from build123d import *

# Parameters (mm, degrees)
ESBO_O1_R                = 2.5
ESBO_O1_R_2              = 7.5
RESSALTO_EXTRUS_O1_DEPTH = 3


with BuildPart() as part:
    # Esboço1 → Ressalto-extrusão1 (new body)
    with BuildSketch(Plane.XY):
        Polygon((40.700385396, -30), (10.700385396, -30), (10.700385396, -33), (-19.299614604, -33), (-19.299614604, -30), (-49.299614604, -30), (-49.299614604, -33), (-79.299614604, -33), (-79.299614604, -30), (-82.299614604, -30), (-82.299614604, -18), (-79.299614604, -18), (-79.299614604, -6), (-82.299614604, -6), (-82.299614604, 6), (-79.299614604, 6), (-79.299614604, 18), (-82.299614604, 18), (-82.299614604, 30), (-79.299614604, 30), (-79.299614604, 33), (-49.299614604, 33), (-49.299614604, 30), (-19.299614604, 30), (-19.299614604, 33), (10.700385396, 33), (10.700385396, 30), (40.700385396, 30), (40.700385396, 33), (70.700385396, 33), (70.700385396, 30), (73.700385396, 30), (73.700385396, 18), (70.700385396, 18), (70.700385396, 6), (73.700385396, 6), (73.700385396, -6), (70.700385396, -6), (70.700385396, -18), (73.700385396, -18), (73.700385396, -30), (70.700385396, -30), (70.700385396, -33), (40.700385396, -33), align=None)
        with Locations((-54.299614604, 0)):
            Circle(ESBO_O1_R, mode=Mode.SUBTRACT)
        with Locations((-29.299614604, 0)):
            Circle(ESBO_O1_R, mode=Mode.SUBTRACT)
        with Locations((-4.299614604, 0)):
            Circle(ESBO_O1_R, mode=Mode.SUBTRACT)
        with Locations((40.700385396, 0)):
            Circle(ESBO_O1_R_2, mode=Mode.SUBTRACT)
    extrude(amount=RESSALTO_EXTRUS_O1_DEPTH)


solid = part.part
The listing builds one solid part. Answer for the finished solid, in the listing's coordinates (mm). A direction names the side the tool comes from. Coordinates: 2 decimals unless noted, no trailing zeros. Loops run counter-clockwise (first coordinate to the right, second up) from the corner with the lowest first, then second, coordinate; pieces in that order, holes last. Notation, with made-up numbers: M -5,67.25 L 17,67.25 A9 ccw 17,80.25 Z; hole C -31.75,84.25 d7. An arc over 180 degrees is marked long. Answer in a Markdown table with one row per item.
1) Find section D-D (y = 12). Determine the outline of the cut face in (x, z), then the cut area to 3 significant figures.
Answers below:
| item | result |
|---|---|
| outline | M -79.3,0 L 70.7,0 L 70.7,3 L -79.3,3 Z |
| area | 450 mm^2 |
2) Given pin 1 (0.9 mm diameter, centred on y = 31.5, z = 1.5, fed in from +X); pin 2 (1.5 mm diameter, centred on x = 72.5, z = 2, fed in from -Y); pin 3 (0.9 mm diameter, centred on x = -81.5, z = 2, fed in from +Y), each flat-ended and moving along its own axis, determine where each tip first touches the part or whether it passes through.
Answers below:
| item | result |
|---|---|
| pin 1 | x = 70.7 |
| pin 2 | y = -30 |
| pin 3 | y = 30 |
3) Find section C-C (z = 1). Count the separate pieces of the cut face and the enclosed holes in it, then the cut area to 3 significant figures.
Answers below:
| item | result |
|---|---|
| separate pieces | 1 |
| enclosed holes | 4 |
| area | 9,520 mm^2 |
4) Determine the mould class of faces 1 (the flat face through (72, -18, 1)), 2 (the flat face through (10.7, -31, 1)), 3 (the flat face through (-82.3, -24, 1)) for opening direction X: released by +X, released by -X, zero draft, split by the parting line, or undercut.
Answers below:
| item | result |
|---|---|
| face 1 | zero draft |
| face 2 | undercut |
| face 3 | released by -X |
5) Find section B-B (x = -45). Determine the outline of the cut face in (y, z).
Answers below:
| item | result |
|---|---|
| outline | M -30,0 L 30,0 L 30,3 L -30,3 Z |
6) Find the intervals of material crossed by probe 1 along X at (y, z) = (12, 1.5); probe 2 along Y at (x, z) = (23, 1.6); probe 3 along X at (y, z) = (3, 0.9), in increasing order.
Answers below:
| item | result |
|---|---|
| probe 1 | -79.3 to 70.7 |
| probe 2 | -30 to 30 |
| probe 3 | -82.3 to 33.83, 47.57 to 73.7 |
7) Which of the six approach directions +Z, -Z, +X, -X, +Y, -Y give full straight-line access (tool end or side, diameter ignored) to faces 4 (the flat face through (72, -6, 1)), 5 (the flat face through (-81, 18, 1)), 6 (the flat face through (-19.3, 31, 1))?
Answers below:
| item | result |
|---|---|
| face 4 | +Z, -Z, +X |
| face 5 | +Z, -Z, -X |
| face 6 | +Z, -Z, +Y |
8) Find section A-A (y = 0). Determine the outline of the cut face in (x, z).
Answers below:
| item | result |
|---|---|
| outline | M -82.3,0 L -56.8,0 L -56.8,3 L -82.3,3 Z; M -51.8,0 L -31.8,0 L -31.8,3 L -51.8,3 Z; M -26.8,0 L -6.8,0 L -6.8,3 L -26.8,3 Z; M -1.8,0 L 33.2,0 L 33.2,3 L -1.8,3 Z; M 48.2,0 L 73.7,0 L 73.7,3 L 48.2,3 Z |
